The listing builds one solid part. Answer for the finished solid, in the listing's coordinates (mm). A direction names the side the tool comes from. Give positions to 0.01 mm unless a question says otherwise; leave off trailing zeros. Order: outer loops, then holes, each group sorted by start corner. A loop starts at its lowest first (then second) coordinate and runs counter-clockwise, first axis right, second up. Notation, with made-up numbers: (9.25, -27) - (37.25, -27) arc R8 cw to (37.25, -18) - close; hole circle Ø7 at (29, 81). An arc over 180 degrees is marked (long way). Use a Markdown table: item, result. Add a question column.
1) The mould has two halves that part along Y. Classify faces 5 (the face through (0, 0, 11.43)), 6 (the face through (-1, 0, -1)), 7 (the face through (-0.509, -2.294, 7.567)): released by +Y, released by -Y, zero draft, split by the parting line, or undercut.
2) Find section D-D, the plane x = -9.5. Determine the outline of the cut face in (y, z), plus the area to 3 significant figures.
3) Flat-ended cylindrical pins translate along their axes: pin 1 (5 mm diameter, centred on y = 6.5, z = 2.5, fed in from +X); pin 2 (1 mm diameter, centred on x = 8, y = 5, fed in from -Z); pin 3 (0.6 mm diameter, centred on x = -1, z = -0.5, fed in from +Y). Find the tip coordinate at first contact, or state that the pin passes through.
4) For faces 1 (the face through (1, 0, 0)), 2 (the face through (-1.6, 8.713, -0.3)), 3 (the face through (-1.7, -9.067, -0.3)), 4 (the face through (0, -5, 2.54)), determine the directions among +Z, -Z, +X, -X, +Y, -Y from which every point of the face is accessible in a straight line to the end or side of a thin tool.
5) Straight lines are drawn through the part: line 1 (Z direction, x = 9, y = 4.75); line 2 (Z direction, x = 0.5, y = 0.75); line 3 (Y direction, x = -0.5, z = 0.5). For each, find the intervals that lie inside material, in ascending order.
6) Find section A-A, the plane z = 0.5. Determine the outline of the cut face in (x, y).
7) Find section C-C, the plane z = 8. Determine the outline of the cut face in (x, y).
8) Find section B-B, the plane x = -5. Determine the outline of the cut face in (y, z).
from build123d import *

# Parameters (mm, degrees)
F0_R     = 2.35
F1_DEPTH = 11.43
F0_R_2   = 4.636
F2_DEPTH = 3.81
F0_R_3   = 11
F3_DEPTH = 2.54
F5_DEPTH = 1.27
F6_SIZE  = 1.26999
F7_R     = 1.26999


# Not quite as in the source:
# - a fillet or chamfer is up to 0.001 mm smaller than in the source, because OpenCascade refuses the exact size


with BuildPart() as f1:
    # F0 (on Top) → F1 (new body)
    with BuildSketch(Plane.XY):
        Circle(F0_R)
    extrude(amount=F1_DEPTH)

    # F0 (on Top) → F2 (join)
    with BuildSketch(Plane.XY):
        Circle(F0_R_2)
        Circle(F0_R, mode=Mode.SUBTRACT)
    extrude(amount=F2_DEPTH)

    # F0 (on Top) → F3 (join)
    with BuildSketch(Plane.XY):
        Circle(F0_R_3)
        Circle(F0_R_2, mode=Mode.SUBTRACT)
    extrude(amount=F3_DEPTH)

    # F4 (on face) → F5 (join)
    with BuildSketch(Plane.XY):
        with BuildLine():
            ThreePointArc((0, 5.4110168739), (3.4329052601, -0.1769831261), (0, -5.7649831261))
            Line((0, -5.7649831261), (0, -9.0669831261))
            ThreePointArc((0, -9.0669831261), (6.8902932862, -0.1769831261), (0, 8.7130168739))
            Line((0, 8.7130168739), (0, 5.4110168739))
        make_face()
        Polygon((0, -9.0669831261), (0, -5.7649831261), (0, 5.4110168739), (0, 8.7130168739), (-3.302, 8.7130168739), (-3.302, -9.0669831261), align=None)
    extrude(amount=-F5_DEPTH)

    # F6 (size 1.27 in the source; OpenCascade refuses exactly that, so slightly less here)
    f6_edges = [f1.edges().sort_by_distance(p)[0] for p in [
        (-3.302, -0.176983, -1.27),
        (0, -0.176983, -1.27),
    ]]
    chamfer(f6_edges, length=F6_SIZE)

    # F7 (radius 1.27 in the source; OpenCascade refuses exactly that, so slightly less here)
    f7_edges = [f1.edges().sort_by_distance(p)[0] for p in [
        (6.890293, -0.176983, -1.27),
    ]]
    fillet(f7_edges, radius=F7_R)


solid = f1.part
The answers:
| question | item | result |
|---|---|---|
| 1 | face 5 | zero draft |
| 1 | face 6 | undercut |
| 1 | face 7 | split by the parting line |
| 2 | outline | (-5.55, 0) - (5.55, 0) - (5.55, 2.54) - (-5.55, 2.54) - close |
| 2 | area | 28.2 mm2 |
| 3 | pin 1 | x = 10.25 |
| 3 | pin 2 | z = 0 |
| 3 | pin 3 | y = 8.71 |
| 4 | face 1 | -Z |
| 4 | face 2 | -Z, +X, -X, +Y |
| 4 | face 3 | -Z, +X, -X, -Y |
| 4 | face 4 | +Z |
| 5 | line 1 | 0 to 2.54 |
| 5 | line 2 | 0 to 11.43 |
| 5 | line 3 | -10.99 to 10.99 |
| 6 | outline | circle Ø22 at (0, 0) |
| 7 | outline | circle Ø4.7 at (0, 0) |
| 8 | outline | (-9.8, 0) - (9.8, 0) - (9.8, 2.54) - (-9.8, 2.54) - close |
